Part model, mm, in its own coordinate system. Face numbers are marked on the shaded views. A direction names the side the tool comes from. Coordinates: 2 decimals unless noted, no trailing zeros. Write each loop counter-clockwise with the first axis right and the second up, starting at its lowest first coordinate (ties: lowest second). Pieces come first, ordered by that corner, then holes. Notation, with made-up numbers: (15, 65) -> (30, 65) arc R10 ccw to (30, 72) -> close; hole circle Ø3 at (-14.5, 31). An arc over 180 degrees is marked (long way). One line per question, with ' | ' between items. Start each with the question number.
Item 1: Probe probe 1 along X at (y, z) = (1.5, -1); probe 2 along X at (y, z) = (-3.5, 5); probe 3 along Y at (x, z) = (84.5, -0.25). List the from-to ranges inside material, lowest first. Write a range as [from, to].
Item 2: Saw through at D-D (y = -12). List the corners of the cut face in (x, z).
Item 3: Pin check, flat tips, straight feed: pin 1 (1 mm diameter, centred on y = 0, z = 2, fed in from -X); pin 2 (0.9 mm diameter, centred on y = 3, z = -0.5, fed in from +X); pin 3 (0.9 mm diameter, centred on y = 2.5, z = -0.5, fed in from -X); pin 4 (1.5 mm diameter, centred on x = 68, z = 1.5, fed in from -Y). Stop position of each tip, or through.
Item 4: Saw through at A-A (y = 0). List the corners of the cut face in (x, z).
Item 5: Saw through at C-C (x = 16). List the corners of the cut face in (y, z).
Item 6: 3-axis set-ups, long thin cutter, end or side, ignore diameter. For the marked faces 1, 2 and 3: which of +Z, -Z, +X, -X, +Y, -Y reach the whole face in a straight line?
Item 7: Saw through at B-B (z = 0). List the corners of the cut face in (x, y), and give its area (3 significant figures).
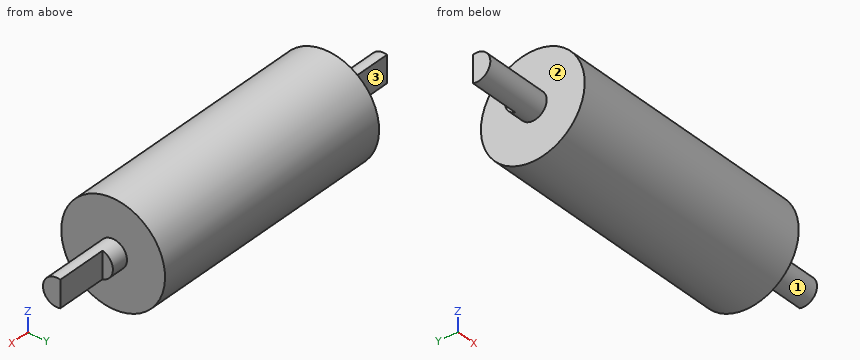
from build123d import *

# Parameters (mm, degrees)
ESBO_O8_R                = 4
RESSALTO_EXTRUS_O4_DEPTH = 20
ESBO_O9_R                = 15
RESSALTO_EXTRUS_O5_DEPTH = 76
ESBO_O10_R               = 4
RESSALTO_EXTRUS_O6_DEPTH = 20
ESBO_O11_W               = 14.978284248
ESBO_O11_H               = 3
CORTE_EXTRUS_O1_DEPTH    = 15
ESBO_O12_W               = 14.281633968
ESBO_O12_H               = 3
CORTE_EXTRUS_O2_DEPTH    = 15


with BuildPart() as part:
    # Esboço8 → Ressalto-extrusão4 (new body)
    with BuildSketch(Plane(origin=(0, 0, 0), x_dir=(0, 0, -1), z_dir=(1, 0, 0))):
        Circle(ESBO_O8_R)
    extrude(amount=RESSALTO_EXTRUS_O4_DEPTH)

    # Esboço9 → Ressalto-extrusão5 (add)
    with BuildSketch(Plane(origin=(20, 0, 0), x_dir=(0, 0, -1), z_dir=(1, 0, 0))):
        Circle(ESBO_O9_R)
    extrude(amount=RESSALTO_EXTRUS_O5_DEPTH)

    # Esboço10 → Ressalto-extrusão6 (add)
    with BuildSketch(Plane(origin=(96, 0, 0), x_dir=(0, 0, -1), z_dir=(1, 0, 0))):
        Circle(ESBO_O10_R)
    extrude(amount=RESSALTO_EXTRUS_O6_DEPTH)

    # Esboço11 → Corte-extrusão1 (cut)
    with BuildSketch(Plane.ZY):
        with Locations((-0.140546903, 2.5)):
            Rectangle(ESBO_O11_W, ESBO_O11_H)
    extrude(amount=-CORTE_EXTRUS_O1_DEPTH, mode=Mode.SUBTRACT)

    # Esboço12 → Corte-extrusão2 (cut)
    with BuildSketch(Plane(origin=(116, 0, 0), x_dir=(0, 0, -1), z_dir=(1, 0, 0))):
        with Locations((0.158049163, 2.5)):
            Rectangle(ESBO_O12_W, ESBO_O12_H)
    extrude(amount=-CORTE_EXTRUS_O2_DEPTH, mode=Mode.SUBTRACT)


solid = part.part
From the geometry:
1) probe 1: [15, 101] | probe 2: [20, 96] | probe 3: [-15, 15]
2) outline: (20, -9) -> (96, -9) -> (96, 9) -> (20, 9) -> close
3) pin 1: x = 0 | pin 2: x = 101 | pin 3: x = 15 | pin 4: y = -14.98
4) outline: (0, -4) -> (20, -4) -> (20, -15) -> (96, -15) -> (96, -4) -> (116, -4) -> (116, 4) -> (96, 4) -> (96, 15) -> (20, 15) -> (20, 4) -> (0, 4) -> close
5) outline: circle Ø8 at (0, 0)
6) face 1: +X | face 2: -X | face 3: +Z, -Z, -X, +Y
7) outline: (0, -4) -> (20, -4) -> (20, -15) -> (96, -15) -> (96, -4) -> (116, -4) -> (116, 1) -> (101, 1) -> (101, 4) -> (96, 4) -> (96, 15) -> (20, 15) -> (20, 4) -> (15, 4) -> (15, 1) -> (0, 1) -> close | area: 2,510 mm2
